For this review, use the dimensioned drawing (mm, ordinates from the lowest corner) and the shaded views. A direction names the side the tool comes from. Round coordinates to 2 decimals unless told otherwise and drop trailing zeros. Write each loop counter-clockwise with the first axis right and the second up, starting at its lowest first coordinate (ties: lowest second). Pieces come first, ordered by that corner, then holes.
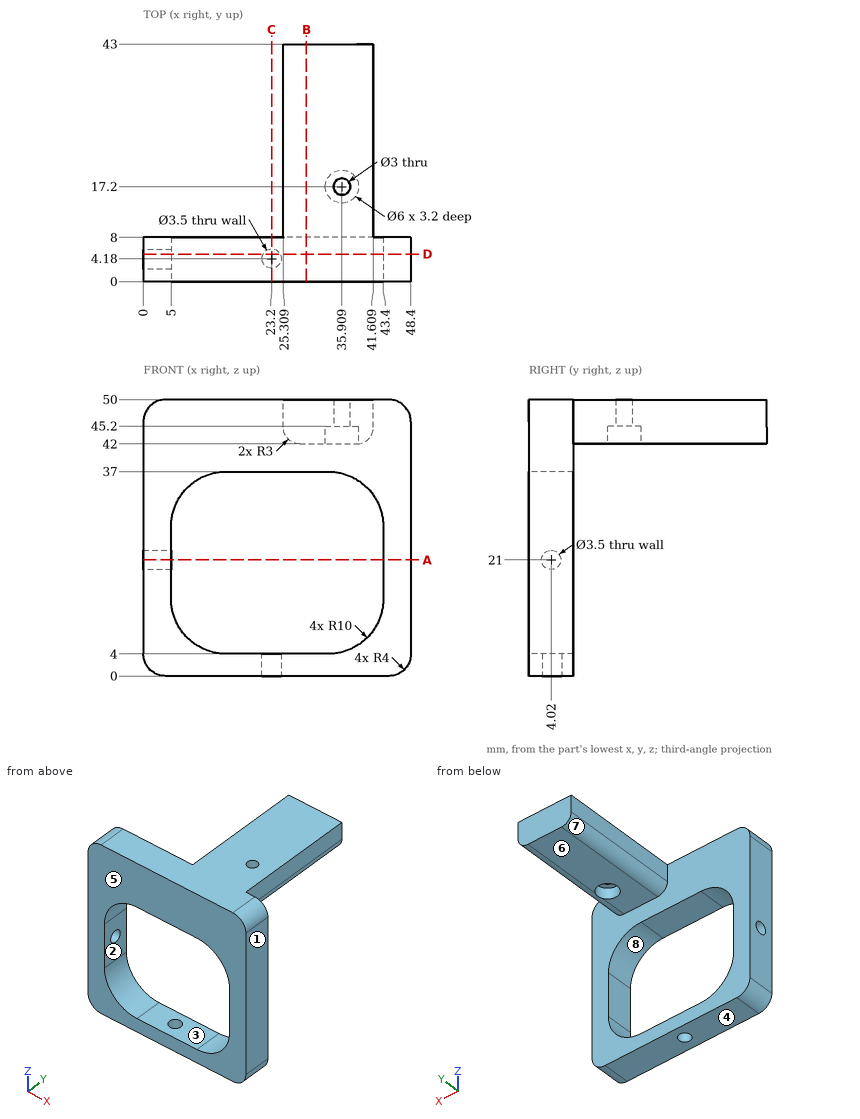
(1) Mouldability with a two-part tool opening along X and no side actions: class the marked faces 1, 2, 3 and 4 as pulls with the +X half, pulls with the -X half, needs draft (parallel to the pull), parting line crosses it, or undercut.
Geometry check:
face 1: pulls with the +X half
face 2: undercut
face 3: undercut
face 4: needs draft
(2) We need section C-C, the plane x = 23.2. Give the boundary of the cut face in (y, z).
Geometry check:
outline: (0, 0) - (2.43, 0) - (2.43, 4) - (0, 4) - close; (0, 37) - (8, 37) - (8, 50) - (0, 50) - close; (5.93, 0) - (8, 0) - (8, 4) - (5.93, 4) - close
(3) We need section D-D, the plane y = 5. Give the boundary of the cut face in (x, z).
Geometry check:
outline: (0, 4) arc R4 ccw to (4, 0) - (21.65, 0) - (21.65, 4) - (15, 4) arc R10 cw to (5, 14) - (5, 19.55) - (0, 19.55) - close; (0, 22.45) - (5, 22.45) - (5, 27) arc R10 cw to (15, 37) - (33.4, 37) arc R10 cw to (43.4, 27) - (43.4, 14) arc R10 cw to (33.4, 4) - (24.75, 4) - (24.75, 0) - (44.4, 0) arc R4 ccw to (48.4, 4) - (48.4, 46) arc R4 ccw to (44.4, 50) - (4, 50) arc R4 ccw to (0, 46) - close
(4) For line 1 along Y through (x, z) = (23.2, 1.4); line 2 along Y through (x, z) = (1.65, 21); line 3 along X through (y, z) = (17, 47) (1 decimal), list the stretches that pass through material, from the lowest coordinate up.
Geometry check:
line 1: y = 0 to 2.43, 5.93 to 8
line 2: y = 0 to 2.27, 5.77 to 8
line 3: x = 25.3 to 34.4, 37.4 to 41.6
(5) For the marked faces 5, 6, 7 and 8, list the 3-axis set-ups (+Z, -Z, +X, -X, +Y, -Y) from which the entire face can be reached by the end or side of a thin tool; tool diameter is ignored.
Geometry check:
face 5: +Z, -Z, +X, -X, -Y
face 6: -Z, +X, -X, +Y
face 7: -Z, -X, +Y
face 8: +Y, -Y
(6) For pin 1 Ø14.5 at (x, z) = (30.5, 24) entering from +Y; pin 2 Ø2.5 at (y, z) = (23.5, 46.5) entering from +X; pin 3 Ø8 at (x, y) = (35, 29) entering from -Z; pin 4 Ø2 at (x, y) = (23.2, 4.18) entering from -Z, all flat-tipped, find the tip position at first contact; note any pin that passes through.
Geometry check:
pin 1: passes through
pin 2: stops at x = 41.61
pin 3: stops at z = 42
pin 4: stops at z = 37
(7) We need section A-A, the plane z = 21. Give the boundary of the cut face in (x, y), and give its area (3 significant figures).
Geometry check:
outline: (0, 0) - (5, 0) - (5, 2.27) - (0, 2.27) - close; (0, 5.77) - (5, 5.77) - (5, 8) - (0, 8) - close; (43.4, 0) - (48.4, 0) - (48.4, 8) - (43.4, 8) - close
area: 62.5 mm2
(8) We need section B-B, the plane x = 29.5. Give the boundary of the cut face in (y, z).
Geometry check:
outline: (0, 0) - (8, 0) - (8, 4) - (0, 4) - close; (0, 37) - (8, 37) - (8, 42) - (43, 42) - (43, 50) - (0, 50) - close
